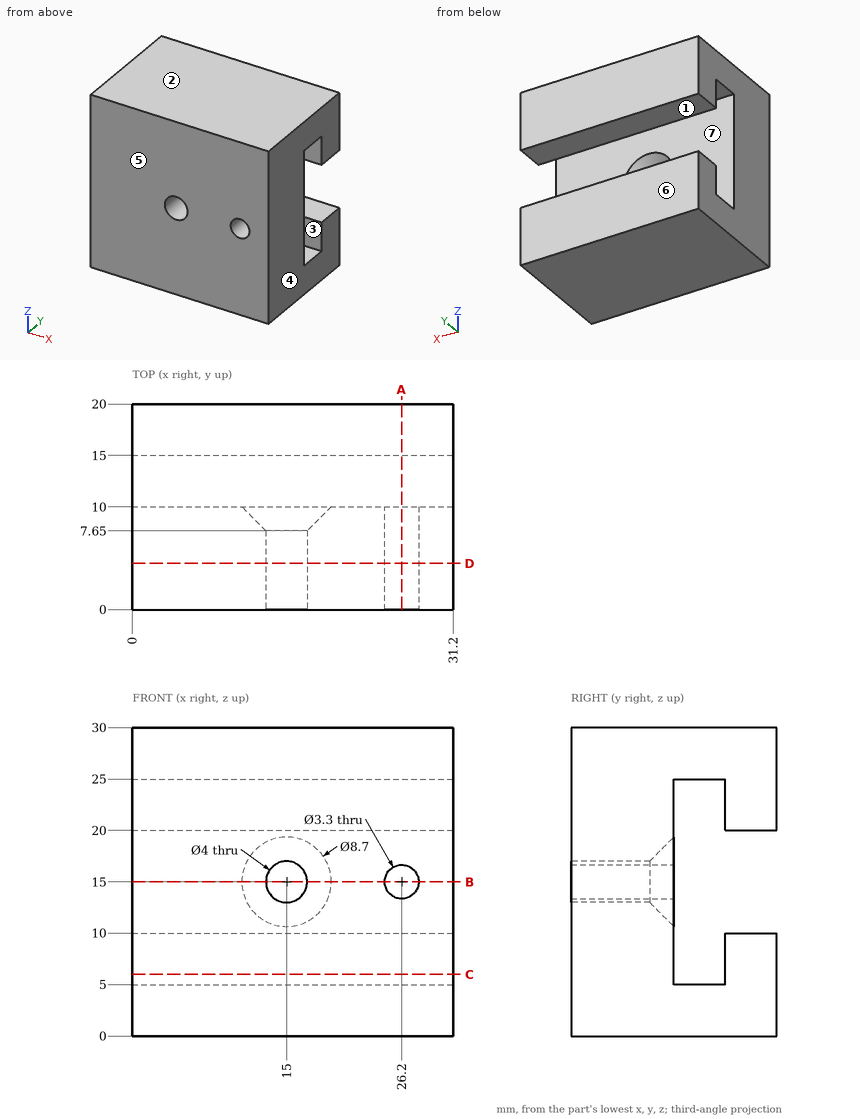
Answer from the drawing. Dimensions are ordinates in mm from the lowest x, y and z of the part. A direction names the side the tool comes from. Round coordinates to 2 decimals unless told otherwise and drop trailing zeros. Loops run counter-clockwise (first coordinate to the right, second up) from the corner with the lowest first, then second, coordinate; pieces in that order, holes last. Notation, with made-up numbers: (-5, 36.5) - (35, 36.5) arc R24 cw to (35, 64.5) - close; hole circle Ø8 at (35, 2). An arc over 180 degrees is marked (long way). Return JSON: item names as keys, results as strings. Group by question number.
1. The part is cut by section C-C on z = 6. Determine the outline of the cut face in (x, y).
2. Consider probe 1 along X at (y, z) = (4, 15); probe 2 along Z at (x, y) = (15, 5); probe 3 along Z at (x, y) = (26.2, 3.25). Determine where each line is inside the solid, lowest interval first.
3. The mould has two halves that part along Y. Classify the marked faces 4, 5, 6 and 7: pulls with the +Y half, pulls with the -Y half, needs draft (parallel to the pull), parting line crosses it, or undercut.
4. The part is cut by section D-D on y = 4.5. Determine the outline of the cut face in (x, z).
5. The part is cut by section A-A on x = 26.2. Determine the outline of the cut face in (y, z).
6. The part is cut by section B-B on z = 15. Determine the outline of the cut face in (x, y).
7. Which of the six approach directions +Z, -Z, +X, -X, +Y, -Y give full straight-line access (tool end or side, diameter ignored) to the marked faces 1, 2 and 3?
8. This flat-tipped pin is pushed along its axis until it touches: P1, Ø3, axis at x = 26.2, z = 15, coming from the -Y side. Where does it stop, or does it pass through?
Resolved:
{
 "1": {"outline": "(0, 0) - (31.2, 0) - (31.2, 10) - (0, 10) - close; (0, 15) - (31.2, 15) - (31.2, 20) - (0, 20) - close"},
 "2": {"probe 1": "x = 0 to 13, 17 to 24.55, 27.85 to 31.2", "probe 2": "z = 0 to 13, 17 to 30", "probe 3": "z = 0 to 13.35, 16.65 to 30"},
 "3": {"face 4": "needs draft", "face 5": "pulls with the -Y half", "face 6": "pulls with the +Y half", "face 7": "undercut"},
 "4": {"outline": "(0, 0) - (31.2, 0) - (31.2, 30) - (0, 30) - close; hole circle Ø4 at (15, 15); hole circle Ø3.3 at (26.2, 15)"},
 "5": {"outline": "(0, 0) - (20, 0) - (20, 10) - (15, 10) - (15, 5) - (10, 5) - (10, 13.35) - (0, 13.35) - close; (0, 16.65) - (10, 16.65) - (10, 25) - (15, 25) - (15, 20) - (20, 20) - (20, 30) - (0, 30) - close"},
 "6": {"outline": "(0, 0) - (13, 0) - (13, 7.65) - (10.65, 10) - (0, 10) - close; (17, 0) - (24.55, 0) - (24.55, 10) - (19.35, 10) - (17, 7.65) - close; (27.85, 0) - (31.2, 0) - (31.2, 10) - (27.85, 10) - close"},
 "7": {"face 1": "+X, -X, +Y", "face 2": "+Z, +X, -X, +Y, -Y", "face 3": "+X, -X"},
 "8": {"P1": "passes through"}
}
